Autodesk Fusion 360 part; units mm, degrees
sketch "Smartie Hopper servo arm" plane through (0, 0, 0) normal (0, 0, 1) x (1, 0, 0)
  circle A0 centre (0, 0) radius 10
  circle A1 centre (0, 0) radius 3.5
  line L0 (-3.25, 25) -> (-3.25, 10)
  line L1 (3.25, 25) -> (3.25, 10)
  line L2 (-7.25, 25) -> (-7.25, 6.8875)
  line L3 (7.25, 25) -> (7.25, 6.8875)
  line L4 (-3.25, 10) -> (3.25, 10)
  line L5 (-7.25, 25) -> (-3.25, 25)
  line L6 (3.25, 25) -> (7.25, 25)
  circle A2 centre (-5.25, 25) radius 2
  circle A3 centre (5.25, 25) radius 2
  dimension "d3" = 7
  dimension "d5" = 20
  dimension "d28" = 3.25
  dimension "d29" = 3.25
  dimension "d34" = 4
  dimension "d35" = 4
  dimension "d36" = 15
  dimension "d37" = 15
  dimension "d38" = 4
  dimension "d39" = 4
extrude "Extrude1" add sketch "Smartie Hopper servo arm" along normal blind 3
fillet "Fillet4" radius 2 2 edges at (3.25, 10, 1.5) (-3.25, 10, 1.5)
fillet "Fillet3" radius 2 2 edges at (7.25, 6.8875, 1.5) (-7.25, 6.8875, 1.5)
equation "stainless_steel_thickness = 3 mm"
equation "arm_thickness = 4 mm"
equation "d10 = stainless_steel_thickness"
equation "groove_diameter = 6.5 mm"
equation "groove_length = 17 mm"
equation "d28 = groove_diameter / 2"
equation "d29 = groove_diameter / 2"
equation "d34 = arm_thickness"
equation "d35 = arm_thickness"
equation "d36 = groove_length - ( arm_thickness / 2 )"
equation "d37 = groove_length - ( arm_thickness / 2 )"
equation "d38 = arm_thickness"
equation "d39 = arm_thickness"
The listing builds one solid part. Answer for the finished solid, in the listing's coordinates (mm). A direction names the side the tool comes from. Give positions to 0.01 mm unless a question says otherwise; leave off trailing zeros. Write each loop counter-clockwise with the first axis right and the second up, starting at its lowest first coordinate (ties: lowest second). Pieces come first, ordered by that corner, then holes. Notation, with made-up numbers: (4.25, -18) -> (30.25, -18) arc R21 ccw to (30.25, 19) -> close; hole circle Ø7 at (74, -5). An arc over 180 degrees is marked (long way). One line per question, with ' | ' between items. Start each with the question number.
1. Given pin 1 Ø0.9 at (y, z) = (19.5, 2) entering from +X; pin 2 Ø1.5 at (x, z) = (-1.5, 1) entering from +Y; pin 3 Ø4 at (x, y) = (0, 0) entering from -Z; pin 4 Ø1.5 at (y, z) = (20.5, 1.5) entering from -X, each flat-ended and moving along its own axis, determine where each tip first touches the part or whether it passes through.
2. Section C-C (y = 23.5) is taken. Determine the outline of the cut face in (x, z), plus the area to 3 significant figures.
3. Section D-D (x = -5.25) is taken. Determine the outline of the cut face in (y, z).
4. For a pull along X with two mould halves and no side action, classify faces 4 (the flat face through (0, 10, 1)), 5 (the cylindrical face through (0, -10, 1)), 6 (the flat face through (-7.25, 16, 1)) as pulls with the +X half, pulls with the -X half, needs draft (parallel to the pull), parting line crosses it, or undercut.
5. For faces 1 (the flat face through (7.25, 16, 1)), 2 (the flat face through (-3.25, 19, 1)), 3 (the cylindrical face through (-7.37, 6.96, 1.52)), determine the directions among +Z, -Z, +X, -X, +Y, -Y from which every point of the face is accessible in a straight line to the end or side of a thin tool.
6. Find the intervals of material crossed by probe 1 along X at (y, z) = (22, 0.5); probe 2 along Y at (x, z) = (0, 1.9); probe 3 along X at (y, z) = (1, 0.9), in increasing order.
7. Section A-A (y = 0) is taken. Determine the outline of the cut face in (x, z), plus the area to 3 significant figures.
8. Section B-B (z = 1) is taken. Determine the outline of the cut face in (x, y), plus the area to 3 significant figures.
Response values:
1) pin 1: x = 7.25 | pin 2: y = 10.27 | pin 3: through | pin 4: x = -7.25
2) outline: (-7.25, 0) -> (-3.25, 0) -> (-3.25, 3) -> (-7.25, 3) -> close; (3.25, 0) -> (7.25, 0) -> (7.25, 3) -> (3.25, 3) -> close | area: 24.0 mm2
3) outline: (-8.51, 0) -> (27, 0) -> (27, 3) -> (-8.51, 3) -> close
4) face 4: undercut | face 5: parting line crosses it | face 6: pulls with the -X half
5) face 1: +Z, -Z, +X, +Y | face 2: +Z, -Z, +Y | face 3: +Z, -Z, -X, +Y
6) probe 1: -7.25 to -3.25, 3.25 to 7.25 | probe 2: -10 to -3.5, 3.5 to 10 | probe 3: -9.95 to -3.35, 3.35 to 9.95
7) outline: (-10, 0) -> (-3.5, 0) -> (-3.5, 3) -> (-10, 3) -> close; (3.5, 0) -> (10, 0) -> (10, 3) -> (3.5, 3) -> close | area: 39.0 mm2
8) outline: (-7.71, 6.37) arc R10 ccw (long way) to (7.71, 6.37) arc R2 cw to (7.25, 7.64) -> (7.25, 25) arc R2 ccw to (3.25, 25) -> (3.25, 12) arc R2 cw to (1.25, 10) -> (-1.25, 10) arc R2 cw to (-3.25, 12) -> (-3.25, 25) arc R2 ccw to (-7.25, 25) -> (-7.25, 7.64) arc R2 cw to start; hole circle Ø7 at (0, 0) | area: 424 mm2
